Can you work these out from the model? Positions are in its coordinate system, mm. Face numbers are marked on the shaded views. A direction names the side the tool comes from. Round coordinates to 2 decimals unless told otherwise and drop trailing zeros. Write each loop counter-clockwise with the first axis right and the second up, starting at its lowest first coordinate (ties: lowest second). Pieces come first, ordered by that corner, then holes.
Q1. If we section it at D-D (z = -3): Please give me the cut outline in (x, y), plus the area to 3 significant figures.
Q2. We'd pull the mould along Y, two halves only. Please class the marked faces 4, 5 and 6: +Y half, -Y half, draft (parallel to the pull), parting line (faces both ways), or undercut.
Q3. For the marked faces 1, 2 and 3, which set-ups out of +Z, -Z, +X, -X, +Y, -Y let a thin tool reach every point of the face, with its end or its side?
Q4. Please list where these lines run through material, in increasing order: line 1 along Z through (x, y) = (7, 1.8); line 2 along X through (y, z) = (1, -4); line 3 along Y through (x, z) = (5, -5.5).
Q5. If we section it at C-C (x = 7): Give the number of separate pieces and of enclosed holes in the cut face, plus the area to 3 significant figures.
Q6. If we section it at A-A (z = -27.5): Please give me the cut outline in (x, y).
Q7. I'm going to push flat-ended pins straight in: pin 1 Ø4 at (x, y) = (3.5, 16.5) entering from +Z; pin 2 Ø1.7 at (x, z) = (5.5, -22.5) entering from +Y; pin 3 Ø3 at (x, z) = (6.5, -19.5) entering from +Y. Where does each tip first touch, or does it pass through?
Q8. If we section it at B-B (y = 40): Please give me the cut outline in (x, z), plus the area to 4 significant figures.
from build123d import *

# Parameters (mm, degrees)
CROQUIS2_W              = 14
CROQUIS2_H              = 31
CROQUIS2_R              = 1.55
SALIENTE_EXTRUIR1_DEPTH = 50
CROQUIS3_W              = 26
CROQUIS3_H              = 45
CORTAR_EXTRUIR1_DEPTH   = 14
CORTAR_EXTRUIR2_DEPTH   = 5
CORTAR_EXTRUIR3_DEPTH   = 1.5
SALIENTE_EXTRUIR3_DEPTH = 14
CROQUIS7_OUTSIDE_W      = 28.094
CROQUIS7_OUTSIDE_H      = 45.094
CORTAR_EXTRUIR5_DEPTH   = 45
REDONDEO1_R             = 2
CROQUIS8_W              = 14
CROQUIS8_H              = 0.5
CORTAR_EXTRUIR6_DEPTH   = 50


with BuildPart() as part:
    # Croquis2 → Saliente-Extruir1 (new body)
    with BuildSketch(Plane(origin=(0, 0, 0), x_dir=(1, 0, 0), z_dir=(0, 1, 0))):
        with Locations((7, 15.5)):
            Rectangle(CROQUIS2_W, CROQUIS2_H)
        with Locations((7, 22)):
            Circle(CROQUIS2_R, mode=Mode.SUBTRACT)
        with Locations((7, 4)):
            Circle(CROQUIS2_R, mode=Mode.SUBTRACT)
    extrude(amount=SALIENTE_EXTRUIR1_DEPTH)

    # Croquis3 → Cortar-Extruir1 (cut)
    with BuildSketch(Plane.ZY):
        with Locations((-13, 27.5)):
            Rectangle(CROQUIS3_W, CROQUIS3_H)
    extrude(amount=-CORTAR_EXTRUIR1_DEPTH, mode=Mode.SUBTRACT)

    # Croquis4 → Cortar-Extruir2 (cut)
    with BuildSketch(Plane(origin=(0, 0, -31), x_dir=(-1, 0, 0), z_dir=(0, 0, -1))):
        with BuildLine():
            Line((-8.55, 8), (-8.55, 18))
            ThreePointArc((-8.55, 18), (-7, 19.55), (-5.45, 18))
            Line((-5.45, 18), (-5.45, 8))
            ThreePointArc((-5.45, 8), (-7, 6.45), (-8.55, 8))
        make_face()
        with BuildLine():
            Line((-8.55, 32), (-8.55, 42))
            ThreePointArc((-8.55, 42), (-7, 43.55), (-5.45, 42))
            Line((-5.45, 42), (-5.45, 32))
            ThreePointArc((-5.45, 32), (-7, 30.45), (-8.55, 32))
        make_face()
    extrude(amount=-CORTAR_EXTRUIR2_DEPTH, mode=Mode.SUBTRACT)

    # Croquis5 → Cortar-Extruir3 (cut)
    with BuildSketch(Plane(origin=(0, 5, 0), x_dir=(1, 0, 0), z_dir=(0, 1, 0))):
        Polygon((10.348631561, 4), (8.674315781, 6.9), (5.325684219, 6.9), (3.651368439, 4), (5.325684219, 1.1), (8.674315781, 1.1), align=None)
        Polygon((8.674315781, 19.1), (10.348631561, 22), (8.674315781, 24.9), (5.325684219, 24.9), (3.651368439, 22), (5.325684219, 19.1), align=None)
    extrude(amount=-CORTAR_EXTRUIR3_DEPTH, mode=Mode.SUBTRACT)

    # Croquis6 → Saliente-Extruir3 (add)
    with BuildSketch(Plane.ZY):
        with BuildLine():
            Line((-26, 5), (-26, 35))
            ThreePointArc((-26, 35), (-20.21590319, 16.698867767), (-5, 5))
            Line((-5, 5), (-26, 5))
        make_face()
    extrude(amount=-SALIENTE_EXTRUIR3_DEPTH)

    # Croquis7 outside → Cortar-Extruir5 (cut)
    with BuildSketch(Plane(origin=(0, 50, 0), x_dir=(1, 0, 0), z_dir=(0, 1, 0))):
        with Locations((7, 15.5)):
            Rectangle(CROQUIS7_OUTSIDE_W, CROQUIS7_OUTSIDE_H)
        Polygon((0, 26), (0, 0), (3, 0), (3, 26), (11, 26), (11, 0), (14, 0), (14, 26), (14, 31), (0, 31), align=None, mode=Mode.SUBTRACT)
    extrude(amount=-CORTAR_EXTRUIR5_DEPTH, mode=Mode.SUBTRACT)

    # Redondeo1
    redondeo1_edges = [part.edges().sort_by_distance(p)[0] for p in [
        (14, 2.5, 0),
        (0, 2.5, 0),
    ]]
    fillet(redondeo1_edges, radius=REDONDEO1_R)

    # Croquis8 → Cortar-Extruir6 (cut)
    with BuildSketch(Plane(origin=(0, 50, 0), x_dir=(1, 0, 0), z_dir=(0, 1, 0))):
        with Locations((7, 30.75)):
            Rectangle(CROQUIS8_W, CROQUIS8_H)
    extrude(amount=-CORTAR_EXTRUIR6_DEPTH, mode=Mode.SUBTRACT)


solid = part.part
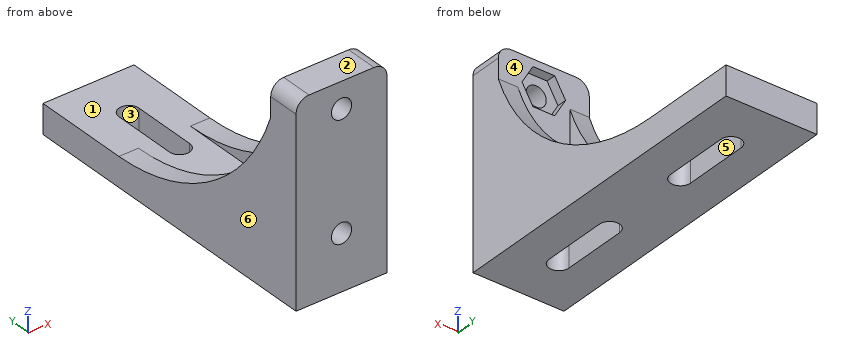
A:
1. outline: (0, 0) - (5.82, 0) - (5.82, 3.5) - (4.23, 3.5) - (4.23, 5) - (0, 5) - close; (8.18, 0) - (14, 0) - (14, 5) - (9.77, 5) - (9.77, 3.5) - (8.18, 3.5) - close
1. area: 53.4 mm2
2. face 4: +Y half
2. face 5: undercut
2. face 6: draft
3. face 1: +Z, +Y
3. face 2: +Z, +X, -X, +Y, -Y
3. face 3: +Z, -Z
4. line 1: z = -30.5 to -23.55, -20.45 to -5.55, -2.45 to 0
4. line 2: x = 0 to 5.45, 8.55 to 14
4. line 3: y = 0 to 3.5
5. separate pieces: 5
5. enclosed holes: 0
5. area: 198 mm2
6. outline: (0, 0) - (14, 0) - (14, 50) - (0, 50) - close; hole (5.45, 8) arc R1.55 ccw to (8.55, 8) - (8.55, 18) arc R1.55 ccw to (5.45, 18) - close; hole (5.45, 32) arc R1.55 ccw to (8.55, 32) - (8.55, 42) arc R1.55 ccw to (5.45, 42) - close
7. pin 1: stops at z = -18.58
7. pin 2: stops at y = 3.5
7. pin 3: stops at y = 5
8. outline: (0, -30.5) - (5.45, -30.5) - (5.45, -26) - (0, -26) - close; (8.55, -30.5) - (14, -30.5) - (14, -26) - (8.55, -26) - close
8. area: 49.05 mm2
